from build123d import *

# Parameters (mm, degrees)
F1_DEPTH = 380
F2_R     = 25
F3_DEPTH = 10
F4_R     = 12.5
F5_DEPTH = 10


with BuildPart() as f1:
    # F0 (on Front) → F1 (new body)
    with BuildSketch(Plane.XZ):
        with BuildLine():
            ThreePointArc((-220, -105), (-205.355339, -140.355339), (-170, -155))
            Line((-170, -155), (170, -155))
            ThreePointArc((170, -155), (205.355339, -140.355339), (220, -105))
            Line((220, -105), (220, 105))
            ThreePointArc((220, 105), (205.355339, 140.355339), (170, 155))
            Line((170, 155), (-170, 155))
            ThreePointArc((-170, 155), (-205.355339, 140.355339), (-220, 105))
            Line((-220, 105), (-220, -105))
        make_face()
        with BuildLine():
            ThreePointArc((195, -105), (187.67767, -122.67767), (170, -130))
            Line((170, -130), (-170, -130))
            ThreePointArc((-170, -130), (-187.67767, -122.67767), (-195, -105))
            Line((-195, -105), (-195, 105))
            ThreePointArc((-195, 105), (-187.67767, 122.67767), (-170, 130))
            Line((-170, 130), (170, 130))
            ThreePointArc((170, 130), (187.67767, 122.67767), (195, 105))
            Line((195, 105), (195, -105))
        make_face(mode=Mode.SUBTRACT)
    extrude(amount=F1_DEPTH)

    # F2 (on face) → F3 (cut)
    with BuildSketch(Plane(origin=(0, 0, -155), x_dir=(1, 0, 0), z_dir=(0, 0, -1))):
        with Locations((-120, 50)):
            Circle(F2_R)
        with Locations((-120, 330)):
            Circle(F2_R)
        with Locations((120, 50)):
            Circle(F2_R)
        with Locations((120, 330)):
            Circle(F2_R)
    extrude(amount=-F3_DEPTH, mode=Mode.SUBTRACT)

    # F4 (on face) → F5 (cut)
    with BuildSketch(Plane.XY.offset(155)):
        with Locations((-120, -50)):
            Circle(F4_R)
        with Locations((-120, -330)):
            Circle(F4_R)
        with Locations((120, -330)):
            Circle(F4_R)
        with Locations((120, -50)):
            Circle(F4_R)
    extrude(amount=-F5_DEPTH, mode=Mode.SUBTRACT)


solid = f1.part
Can you work these out from the model? Positions are in its coordinate system, mm. A direction names the side the tool comes from. Give positions to 0.01 mm unless a question says otherwise; leave off trailing zeros. Write each loop counter-clockwise with the first axis right and the second up, starting at its lowest first coordinate (ties: lowest second). Pieces come first, ordered by that corner, then holes. Notation, with made-up numbers: (36, -28) -> (52, -28) arc R16 cw to (52, -23) -> close; hole circle Ø2 at (-23, -30). An arc over 180 degrees is marked (long way). Answer as a JSON object with one key per item and string values. Group by question number.
Item 1: Suppose I cut it at C-C (y = -240.5). Please give me the cut outline in (x, z), plus the area to 3 significant figures.
Item 2: For faces 5 (the face through (-187.482, -187.34, -122.871)), 6 (the face through (-120, -330, -145)), 7 (the face through (120, -50, 145)), which set-ups out of +Z, -Z, +X, -X, +Y, -Y let a thin tool reach every point of the face, with its end or its side?
Item 3: Suppose I cut it at D-D (x = 32.5). Please give me the cut outline in (y, z), plus the area to 3 significant figures.
Item 4: I'm going to push a flat-ended pin straight in: P1, Ø25, axis at x = -129.5, y = -322, coming from the -Z side. Where does the tip first touch, or does it pass through?
Item 5: We'd pull the mould along X, two halves only. Please class faces 1 (the face through (-120, -50, 145)), 2 (the face through (-204.964, -187.34, 140.742)), 3 (the face through (-17, -380, -137)), 4 (the face through (195, -187, 1)): +X half, -X half, draft (parallel to the pull), parting line (faces both ways), or undercut.
Item 6: Suppose I cut it at A-A (z = 28.5). Please give me the cut outline in (x, y), plus the area to 3 significant figures.
Item 7: Please list where these lines run through material, in increasing order: line 1 (Y direction, x = -120, z = 152); line 2 (Y direction, x = 120, z = -152.5); line 3 (X direction, y = -33, z = 56). Write a range as [from, to].
Item 8: Suppose I cut it at B-B (x = 120). Please give me the cut outline in (y, z), plus the area to 3 significant figures.
Findings:
{
 "1": {"outline": "(-220, -105) arc R50 ccw to (-170, -155) -> (170, -155) arc R50 ccw to (220, -105) -> (220, 105) arc R50 ccw to (170, 155) -> (-170, 155) arc R50 ccw to (-220, 105) -> close; hole (-195, -105) arc R25 ccw to (-170, -130) -> (170, -130) arc R25 ccw to (195, -105) -> (195, 105) arc R25 ccw to (170, 130) -> (-170, 130) arc R25 ccw to (-195, 105) -> close", "area": "33,400 mm²"},
 "2": {"face 5": "+Y, -Y", "face 6": "-Z", "face 7": "+Z"},
 "3": {"outline": "(-380, -155) -> (0, -155) -> (0, -130) -> (-380, -130) -> close; (-380, 130) -> (0, 130) -> (0, 155) -> (-380, 155) -> close", "area": "19,000 mm²"},
 "4": {"P1": "stops at z = -145"},
 "5": {"face 1": "undercut", "face 2": "-X half", "face 3": "draft", "face 4": "undercut"},
 "6": {"outline": "(-220, -380) -> (-195, -380) -> (-195, 0) -> (-220, 0) -> close; (195, -380) -> (220, -380) -> (220, 0) -> (195, 0) -> close", "area": "19,000 mm²"},
 "7": {"line 1": "y = [-380, -342.5], [-317.5, -62.5], [-37.5, 0]", "line 2": "y = [-380, -355], [-305, -75], [-25, 0]", "line 3": "x = [-220, -195], [195, 220]"},
 "8": {"outline": "(-380, -155) -> (-355, -155) -> (-355, -145) -> (-305, -145) -> (-305, -155) -> (-75, -155) -> (-75, -145) -> (-25, -145) -> (-25, -155) -> (0, -155) -> (0, -130) -> (-380, -130) -> close; (-380, 130) -> (0, 130) -> (0, 155) -> (-37.5, 155) -> (-37.5, 145) -> (-62.5, 145) -> (-62.5, 155) -> (-317.5, 155) -> (-317.5, 145) -> (-342.5, 145) -> (-342.5, 155) -> (-380, 155) -> close", "area": "17,500 mm²"}
}
